Input: part model. Units: mm. Frame: model coordinates. A direction names the side the tool comes from. Coordinates: 2 decimals unless noted, no trailing zeros. Loops run counter-clockwise (first coordinate to the right, second up) from the corner with the lowest first, then second, coordinate; pieces in that order, holes last.
Item 1: Section A-A on y = 1.5. Return loops of the section in (x, z).
Item 2: Section C-C on x = 4.5. Return loops of the section in (y, z), and give its area (3 significant figures).
Item 3: Reachability of faces 1 (the flat face through (6.862, 2, 12)), 2 (the flat face through (-4, -13, 14)), 3 (the cylindrical face through (-2.92, -12.01, 6.9)), 4 (the flat face through (6.862, 2, 2)) from +Z, -Z, +X, -X, +Y, -Y: full face, straight path, thin tool, end or side. Return the list, or none.
Item 4: Pull-direction query (X, two-part tool) for faces 5 (the flat face through (-16, 6.057, 7)), 6 (the flat face through (-13.138, 2, 12)), 7 (the flat face through (-13.138, 2, 2)), 8 (the flat face through (14.162, -7, 7)); classes: released by +X, released by -X, zero draft, split by the parting line, or undercut.
Item 5: Ray query, line 1 along X through (y, z) = (3, 0.75); line 2 along X through (y, z) = (-5, 5.75); line 3 along Y through (x, z) = (-4, 5.25). Return the intervals inside material, ascending.
Item 6: Section D-D on z = 8.5. Return loops of the section in (x, y).
```python
from build123d import *

# Parameters (mm, degrees)
F0_W     = 35
F0_H     = 26
F1_DEPTH = 14
F3_DEPTH = 32.63313
F4_R     = 3.95
F5_DEPTH = 25


with BuildPart() as f1:
    # F0 (on Top) → F1 (new body)
    with BuildSketch(Plane.XY):
        with Locations((-3.3376533666, -6.9431716278)):
            Rectangle(F0_W, F0_H)
    extrude(amount=F1_DEPTH)

    # F2 (on face) → F3 (cut)
    with BuildSketch(Plane(origin=(0, 0, 0), x_dir=(1, 0, 0), z_dir=(0, 0, -1))):
        with BuildLine():
            Line((-13.1376533666, 2.1359970383), (-13.1376533666, -6.0568283722))
            Line((-13.1376533666, -6.0568283722), (-8.6545346445, -6.0568283722))
            ThreePointArc((-8.6545346445, -6.0568283722), (-11.8568708771, -2.5044354035), (-13.0148172936, 2.1359970383))
            Line((-13.0148172936, 2.1359970383), (-13.1376533666, 2.1359970383))
        make_face()
        with BuildLine():
            ThreePointArc((-13.0148172936, 2.1359970383), (-11.8568708771, -2.5044354035), (-8.6545346445, -6.0568283722))
            Line((-8.6545346445, -6.0568283722), (2.3792279113, -6.0568283722))
            ThreePointArc((2.3792279113, -6.0568283722), (5.5815641438, -2.5044354035), (6.7395105604, 2.1359970383))
            Line((6.7395105604, 2.1359970383), (-13.0148172936, 2.1359970383))
        make_face()
        with BuildLine():
            ThreePointArc((6.7395105604, 2.1359970383), (5.5815641438, -2.5044354035), (2.3792279113, -6.0568283722))
            Line((2.3792279113, -6.0568283722), (6.8623466334, -6.0568283722))
            Line((6.8623466334, -6.0568283722), (6.8623466334, 2.1359970383))
            Line((6.8623466334, 2.1359970383), (6.7395105604, 2.1359970383))
        make_face()
        with BuildLine():
            ThreePointArc((6.7395105604, 2.1359970383), (-3.1376533666, 12.0131609653), (-13.0148172936, 2.1359970383))
            Line((-13.0148172936, 2.1359970383), (6.7395105604, 2.1359970383))
        make_face()
    extrude(amount=-F3_DEPTH, mode=Mode.SUBTRACT)

    # F4 (on face) → F5 (join)
    with BuildSketch(Plane(origin=(0, 6.0568283722, 0), x_dir=(-1, 0, 0), z_dir=(0, 1, 0))):
        with Locations((13.3731277149, 7)):
            Circle(F4_R)
        with BuildLine():
            ThreePointArc((-6.8623466334, 3.05), (-4.0692748477, 4.2069282143), (-2.9123466334, 7))
            ThreePointArc((-2.9123466334, 7), (-4.0692748477, 9.7930717857), (-6.8623466334, 10.95))
            Line((-6.8623466334, 10.95), (-6.8623466334, 3.05))
        make_face()
    extrude(amount=-F5_DEPTH)


solid = f1.part
```
Results found:
1. outline: (-20.84, 0) - (-13.14, 0) - (-13.14, 3.06) arc R3.95 ccw to (-13.14, 10.94) - (-13.14, 14) - (-20.84, 14) - close; (6.86, 0) - (14.16, 0) - (14.16, 14) - (6.86, 14) - (6.86, 10.95) arc R3.95 ccw to (6.86, 3.05) - close
2. outline: (-19.94, 0) - (-8.4, 0) - (-8.4, 3.83) - (6.06, 3.83) - (6.06, 10.17) - (-8.4, 10.17) - (-8.4, 14) - (-19.94, 14) - close
2. area: 253 mm2
3. face 1: +Z, +Y
3. face 2: +Z, +X, -X, +Y, -Y
3. face 3: +Y
3. face 4: -Z, +Y
4. face 5: zero draft
4. face 6: undercut
4. face 7: undercut
4. face 8: released by +X
5. line 1: x = -20.84 to -13.14, 6.86 to 14.16
5. line 2: x = -20.84 to -9.63, 3.12 to 14.16
5. line 3: y = -19.94 to -11.98
6. outline: (-20.84, -19.94) - (14.16, -19.94) - (14.16, 6.06) - (3.21, 6.06) - (3.21, -9.7) arc R9.88 cw to (-9.72, -9.5) - (-9.72, 6.06) - (-20.84, 6.06) - close
